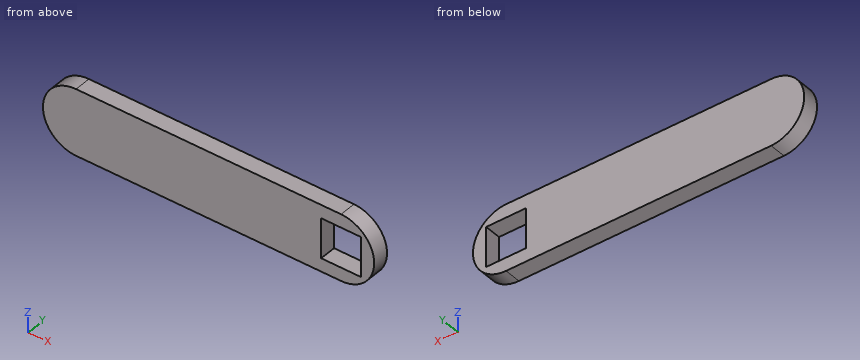
```python
from build123d import *

# Parameters (mm, degrees)
EXTRUDE_1_DEPTH     = 25
SKETCH_3_W          = 60
SKETCH_3_H          = 60
CUT_EXTRUDE_1_DEPTH = 25


with BuildPart() as part:
    # 草图1 → 凸台-拉伸1 (new body)
    with BuildSketch(Plane(origin=(0, 0, 0), x_dir=(1, 0, 0), z_dir=(0, 1, 0))):
        with BuildLine():
            Line((-200, 50), (200, 50))
            ThreePointArc((200, 50), (250, 0), (200, -50))
            Line((200, -50), (-200, -50))
            ThreePointArc((-200, -50), (-250, 0), (-200, 50))
        make_face()
    extrude(amount=EXTRUDE_1_DEPTH)

    # 草图3 → 切除-拉伸1 (cut)
    with BuildSketch(Plane.XZ):
        with Locations((200, 0)):
            Rectangle(SKETCH_3_W, SKETCH_3_H)
    extrude(amount=-CUT_EXTRUDE_1_DEPTH, mode=Mode.SUBTRACT)


solid = part.part
```
For this review, take the finished solid that the model builds, in its own axes (mm). Coordinates: 2 decimals unless noted, no trailing zeros. Order: outer loops, then holes, each group sorted by start corner. A loop starts at its lowest first (then second) coordinate and runs counter-clockwise, first axis right, second up. Notation, with made-up numbers: (47.5, 20) - (80.5, 20) arc R8 cw to (80.5, 31) - close; hole circle Ø3 at (35.5, 61.25). An arc over 180 degrees is marked (long way). Answer as a JSON object with one key per item and string values. Group by question number.
1. We need section C-C on z = 39. State the section outline as (x, y) points, then the cut area to 3 significant figures.
2. We need section A-A on z = 0. State the section outline as (x, y) points.
3. We need section B-B on y = 11. State the section outline as (x, z) points.
4. For probe 1 along X at (y, z) = (17.25, -4); probe 2 along X at (y, z) = (6.75, -20); probe 3 along X at (y, z) = (20.25, -41.5), list the stretches that pass through material, from the lowest coordinate up.
5. Clearance check with flat-ended pins moving along their axes: P1, Ø12.5, axis at y = 11, z = -0.5, coming from the -X side; P2, Ø10, axis at y = 16.5, z = -8, coming from the +X side. State where each tip first meets the part, or that it passes through.
Final values:
{
 "1": {"outline": "(-231.29, 0) - (231.29, 0) - (231.29, 25) - (-231.29, 25) - close", "area": "11,600 mm²"},
 "2": {"outline": "(-250, 0) - (170, 0) - (170, 25) - (-250, 25) - close; (230, 0) - (250, 0) - (250, 25) - (230, 25) - close"},
 "3": {"outline": "(-200, -50) - (200, -50) arc R50 ccw to (200, 50) - (-200, 50) arc R50 ccw to start; hole (170, -30) - (230, -30) - (230, 30) - (170, 30) - close"},
 "4": {"probe 1": "-249.84 to 170, 230 to 249.84", "probe 2": "-245.83 to 170, 230 to 245.83", "probe 3": "-227.89 to 227.89"},
 "5": {"P1": "x = -250", "P2": "x = 249.91"}
}
